Source: CAD feature listing. Evaluate the final solid. Frame: model axes, mm. Face numbers are marked on the shaded views. A direction names the side the tool comes from. Round coordinates to 2 decimals unless told otherwise and drop trailing zeros. Loops run counter-clockwise (first coordinate to the right, second up) from the corner with the lowest first, then second, coordinate; pieces in that order, holes last. Notation, with made-up numbers: M 33,4.5 L 84,4.5 A19 cw 84,16.5 Z; hole C 65,-1.5 d1. An arc over 180 degrees is marked long. One line per item, written item: value.
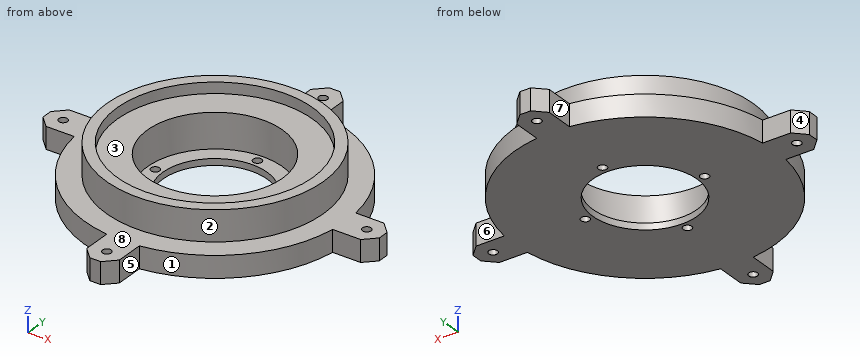
from build123d import *

# Parameters (mm, degrees)
BOSS_EXTRUDE1_DEPTH             = 10
SKETCH2_R                       = 50
BOSS_EXTRUDE2_DEPTH             = 14
SKETCH3_R                       = 31.1
CUT_EXTRUDE1_DEPTH              = 21
F_4_0MM_DOWEL_HOLE1_D           = 4
F_4_0MM_DOWEL_HOLE1_CSINK_D     = 4.05
F_4_0MM_DOWEL_HOLE1_CSINK_ANGLE = 90
SKETCH11_R                      = 45
CUT_EXTRUDE2_DEPTH              = 5
SKETCH4_R                       = 24
CUT_EXTRUDE3_DEPTH              = 4
SKETCH12_R                      = 2
CUT_EXTRUDE5_DEPTH              = 4


with BuildPart() as part:
    # Sketch1 → Boss-Extrude1 (new body)
    with BuildSketch(Plane.XY):
        with BuildLine():
            Line((-42.5, 7.5), (-59.529404499, 7.5))
            ThreePointArc((-59.529404499, 7.5), (-60, 0), (-59.529404499, -7.5))
            Line((-59.529404499, -7.5), (-42.5, -7.5))
            Line((-42.5, -7.5), (-42.5, 7.5))
        make_face()
        with BuildLine():
            ThreePointArc((-7.5, 59.529404499), (-42.426406871, 42.426406871), (-59.529404499, 7.5))
            Line((-59.529404499, 7.5), (-42.5, 7.5))
            Line((-42.5, 7.5), (-42.5, -7.5))
            Line((-42.5, -7.5), (-59.529404499, -7.5))
            ThreePointArc((-59.529404499, -7.5), (-42.426406871, -42.426406871), (-7.5, -59.529404499))
            Line((-7.5, -59.529404499), (-7.5, -42.5))
            Line((-7.5, -42.5), (7.5, -42.5))
            Line((7.5, -42.5), (7.5, -59.529404499))
            ThreePointArc((7.5, -59.529404499), (42.426406871, -42.426406871), (59.529404499, -7.5))
            Line((59.529404499, -7.5), (42.5, -7.5))
            Line((42.5, -7.5), (42.5, 7.5))
            Line((42.5, 7.5), (59.529404499, 7.5))
            ThreePointArc((59.529404499, 7.5), (42.426406871, 42.426406871), (7.5, 59.529404499))
            Line((7.5, 59.529404499), (7.5, 42.5))
            Line((7.5, 42.5), (-7.5, 42.5))
            Line((-7.5, 42.5), (-7.5, 59.529404499))
        make_face()
        with BuildLine():
            ThreePointArc((7.5, 59.529404499), (0, 60), (-7.5, 59.529404499))
            Line((-7.5, 59.529404499), (-7.5, 42.5))
            Line((-7.5, 42.5), (7.5, 42.5))
            Line((7.5, 42.5), (7.5, 59.529404499))
        make_face()
        with BuildLine():
            Line((-7.5, 72.5), (-7.5, 59.529404499))
            ThreePointArc((-7.5, 59.529404499), (0, 60), (7.5, 59.529404499))
            Line((7.5, 59.529404499), (7.5, 72.5))
            Line((7.5, 72.5), (2.5, 77.5))
            Line((2.5, 77.5), (-2.5, 77.5))
            Line((-2.5, 77.5), (-7.5, 72.5))
        make_face()
        with BuildLine():
            Line((-59.529404499, 7.5), (-72.5, 7.5))
            Line((-72.5, 7.5), (-77.5, 2.5))
            Line((-77.5, 2.5), (-77.5, -2.5))
            Line((-77.5, -2.5), (-72.5, -7.5))
            Line((-72.5, -7.5), (-59.529404499, -7.5))
            ThreePointArc((-59.529404499, -7.5), (-60, 0), (-59.529404499, 7.5))
        make_face()
        with BuildLine():
            ThreePointArc((60, 0), (59.882235554, 3.757374753), (59.529404499, 7.5))
            Line((59.529404499, 7.5), (42.5, 7.5))
            Line((42.5, 7.5), (42.5, -7.5))
            Line((42.5, -7.5), (59.529404499, -7.5))
            ThreePointArc((59.529404499, -7.5), (59.882235554, -3.757374753), (60, 0))
        make_face()
        with BuildLine():
            Line((72.5, 7.5), (59.529404499, 7.5))
            ThreePointArc((59.529404499, 7.5), (59.882235554, 3.757374753), (60, 0))
            ThreePointArc((60, 0), (59.882235554, -3.757374753), (59.529404499, -7.5))
            Line((59.529404499, -7.5), (72.5, -7.5))
            Line((72.5, -7.5), (77.5, -2.5))
            Line((77.5, -2.5), (77.5, 2.5))
            Line((77.5, 2.5), (72.5, 7.5))
        make_face()
        with BuildLine():
            ThreePointArc((7.5, -59.529404499), (0, -60), (-7.5, -59.529404499))
            Line((-7.5, -59.529404499), (-7.5, -72.5))
            Line((-7.5, -72.5), (-2.5, -77.5))
            Line((-2.5, -77.5), (2.5, -77.5))
            Line((2.5, -77.5), (7.5, -72.5))
            Line((7.5, -72.5), (7.5, -59.529404499))
        make_face()
        with BuildLine():
            Line((-7.5, -42.5), (-7.5, -59.529404499))
            ThreePointArc((-7.5, -59.529404499), (0, -60), (7.5, -59.529404499))
            Line((7.5, -59.529404499), (7.5, -42.5))
            Line((7.5, -42.5), (-7.5, -42.5))
        make_face()
    extrude(amount=BOSS_EXTRUDE1_DEPTH)

    # Sketch2 → Boss-Extrude2 (add)
    with BuildSketch(Plane.XY.offset(10)):
        Circle(SKETCH2_R)
    extrude(amount=BOSS_EXTRUDE2_DEPTH)

    # Sketch3 → Cut-Extrude1 (cut)
    with BuildSketch(Plane.XY.offset(24)):
        Circle(SKETCH3_R)
    extrude(amount=-CUT_EXTRUDE1_DEPTH, mode=Mode.SUBTRACT)

    # Ø4.0mm Dowel Hole1 (through all)
    with Locations(Plane(origin=(0, 0, 0), x_dir=(-1, 0, 0), z_dir=(0, 0, -1))):
        with Locations((-70, 0), (0, 70), (70, 0), (0, -70)):
            CounterSinkHole(F_4_0MM_DOWEL_HOLE1_D / 2, F_4_0MM_DOWEL_HOLE1_CSINK_D / 2, counter_sink_angle=F_4_0MM_DOWEL_HOLE1_CSINK_ANGLE)

    # Sketch11 → Cut-Extrude2 (cut)
    with BuildSketch(Plane.XY.offset(24)):
        Circle(SKETCH11_R)
    extrude(amount=-CUT_EXTRUDE2_DEPTH, mode=Mode.SUBTRACT)

    # Sketch4 → Cut-Extrude3 (cut)
    with BuildSketch(Plane(origin=(0, 0, 0), x_dir=(-1, 0, 0), z_dir=(0, 0, -1))):
        Circle(SKETCH4_R)
    extrude(amount=-CUT_EXTRUDE3_DEPTH, mode=Mode.SUBTRACT)

    # Sketch12 → Cut-Extrude5 (cut)
    with BuildSketch(Plane(origin=(0, 0, 0), x_dir=(-1, 0, 0), z_dir=(0, 0, -1))):
        with Locations((27.5, 0)):
            Circle(SKETCH12_R)
        with Locations((0, -27.5)):
            Circle(SKETCH12_R)
        with Locations((-27.5, 0)):
            Circle(SKETCH12_R)
        with Locations((0, 27.5)):
            Circle(SKETCH12_R)
    extrude(amount=-CUT_EXTRUDE5_DEPTH, mode=Mode.SUBTRACT)


solid = part.part
1. Ray query, line 1 (Y direction, x = 0, z = 5.75); line 2 (Y direction, x = 70, z = 4.5); line 3 (Y direction, x = 0, z = 18.75). Return the intervals inside material, ascending. Write a range as [from, to].
Report:
line 1: y = [-77.5, -72], [-68, -31.1], [31.1, 68], [72, 77.5]
line 2: y = [-7.5, -2], [2, 7.5]
line 3: y = [-50, -31.1], [31.1, 50]
2. Reachability of the marked faces 5, 6, 7 and 8 from +Z, -Z, +X, -X, +Y, -Y: full face, straight path, thin tool, end or side. Return the list, or none.
Report:
face 5: +Z, -Z, +X, -Y
face 6: +Z, -Z, +X, +Y
face 7: +Z, -Z, -X, +Y
face 8: +Z
3. Section query B-B (y = -70). Return the cut outline in (x, z) (3 decimals).
Report:
outline: M -7.5,0 L -2.025,0 L -2,0.025 L -2,10 L -7.5,10 Z; M 2,0.025 L 2.025,0 L 7.5,0 L 7.5,10 L 2,10 Z
4. Pin query (flat end, axial travel): pin 1 (1 mm diameter, centred on x = 24, y = 26.5, fed in from +Z); pin 2 (5 mm diameter, centred on y = 65.5, z = 2.5, fed in from +X); pin 3 (5 mm diameter, centred on y = 34, z = 17, fed in from -X); pin 4 (2.5 mm diameter, centred on x = 0, y = -27.5, fed in from -Z). Return the tip coordinate at first contact, or that it passes through.
Report:
pin 1: stops at z = 19
pin 2: stops at x = 7.5
pin 3: stops at x = -38.83
pin 4: passes through
5. Section query A-A (z = 8). Count the separate pieces of the cut face and the enclosed holes in it, and give its area (3 significant figures).
Report:
separate pieces: 1
enclosed holes: 5
area: 9,180 mm2
6. Pull-direction query (Y, two-part tool) for the marked faces 1, 2, 3 and 4; classes: released by +Y, released by -Y, zero draft, split by the parting line, or undercut.
Report:
face 1: released by -Y
face 2: split by the parting line
face 3: undercut
face 4: released by +Y
7. Section query D-D (z = 21). Return the cut outline in (x, y).
Report:
outline: C 0,0 d100; hole C 0,0 d90
8. Section query C-C (x = -5.5). Return the cut outline in (y, z), and give its area (3 significant figures).
Report:
outline: M -74.5,0 L -23.36,0 L -23.36,3 L -30.61,3 L -30.61,19 L -44.66,19 L -44.66,24 L -49.7,24 L -49.7,10 L -74.5,10 Z; M 23.36,0 L 74.5,0 L 74.5,10 L 49.7,10 L 49.7,24 L 44.66,24 L 44.66,19 L 30.61,19 L 30.61,3 L 23.36,3 Z
area: 1,320 mm2
